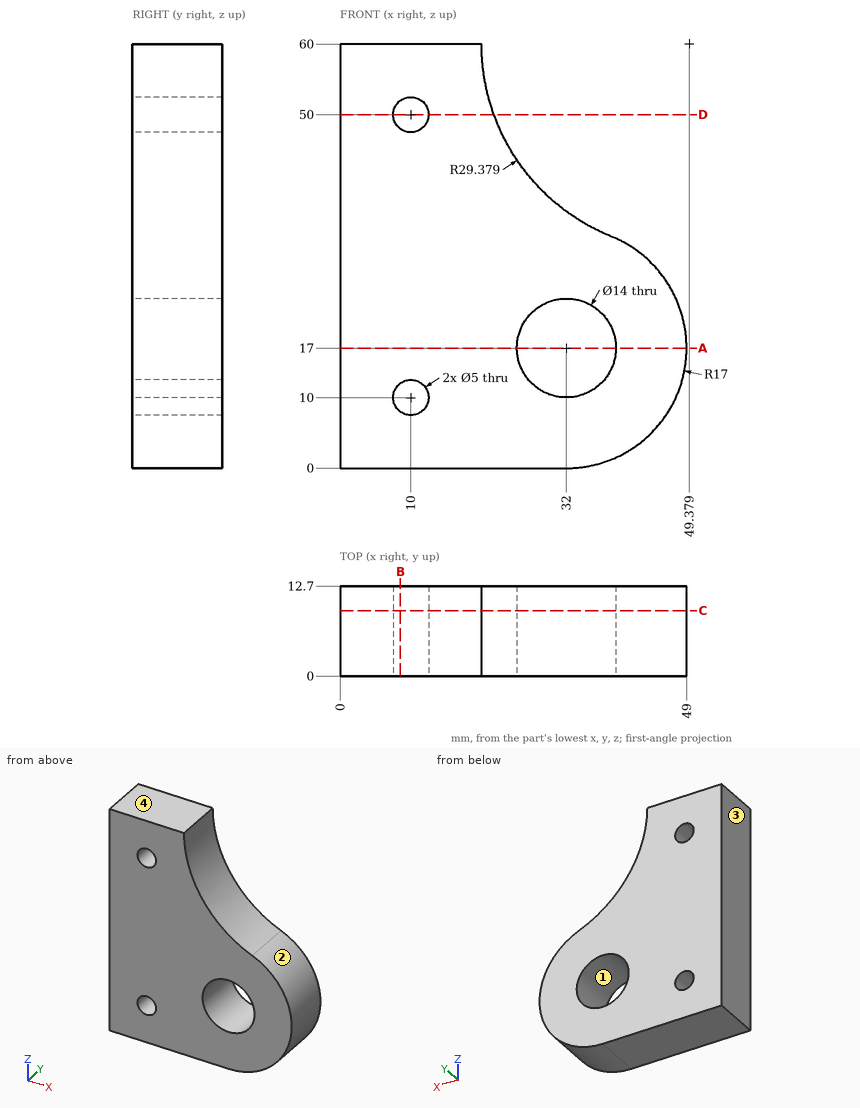
Geometry check sheet. Reference: drawing and pictorial views, mm from the part's lowest x, y, z. Round coordinates to 2 decimals unless told otherwise and drop trailing zeros. Loops run counter-clockwise (first coordinate to the right, second up) from the corner with the lowest first, then second, coordinate; pieces in that order, holes last. Notation, with made-up numbers: M -20,6.5 L 30,6.5 A19 ccw 30,37.5 Z; hole C 89,45 d5. An arc over 180 degrees is marked long. One line per item, written item: value.
(1) Thickness scan on line 1 (X direction, y = 9.75, z = 17); line 2 (Z direction, x = 12, y = 6.75); line 3 (X direction, y = 1.25, z = 8.5). Record the ranges inside material, lowest first.
Computed values:
line 1: x = 0 to 25, 39 to 49
line 2: z = 0 to 8.5, 11.5 to 48.5, 51.5 to 60
line 3: x = 0 to 8, 12 to 46.72
(2) Sectioned sample at D-D, the plane z = 50. Record the cut outline in (x, y).
Computed values:
outline: M 0,0 L 7.5,0 L 7.5,12.7 L 0,12.7 Z; M 12.5,0 L 21.75,0 L 21.75,12.7 L 12.5,12.7 Z
(3) Release check for a two-part mould opening along X. For the marked faces 1, 2, 3 and 4 record: +X half, -X half, draft (parallel to the pull), parting line (faces both ways), or undercut.
Computed values:
face 1: undercut
face 2: +X half
face 3: -X half
face 4: draft
(4) Depth check by flat-ended pin: pin 1 Ø1 at (x, z) = (11.5, 50.5) entering from +Y; pin 2 Ø8 at (x, z) = (10, 10) entering from -Y; pin 3 Ø6 at (y, z) = (4, 43) entering from +X; pin 4 Ø2 at (x, y) = (31.5, 7) entering from +Z. Enter the tip coordinate at first touch or a pass-through.
Computed values:
pin 1: passes through
pin 2: stops at y = 0
pin 3: stops at x = 27.86
pin 4: stops at z = 37.49
(5) Sectioned sample at C-C, the plane y = 9.25. Record the cut outline in (x, z).
Computed values:
outline: M 0,0 L 32,0 A17 ccw 38.37,32.76 A29.38 cw 20,60 L 0,60 Z; hole C 10,10 d5; hole C 10,50 d5; hole C 32,17 d14
(6) Sectioned sample at A-A, the plane z = 17. Record the cut outline in (x, y).
Computed values:
outline: M 0,0 L 25,0 L 25,12.7 L 0,12.7 Z; M 39,0 L 49,0 L 49,12.7 L 39,12.7 Z
(7) Sectioned sample at B-B, the plane x = 8.5. Record the cut outline in (y, z).
Computed values:
outline: M 0,0 L 12.7,0 L 12.7,8 L 0,8 Z; M 0,12 L 12.7,12 L 12.7,48 L 0,48 Z; M 0,52 L 12.7,52 L 12.7,60 L 0,60 Z
